from build123d import *

# Parameters (mm, degrees)
BOSS_EXTRUDE1_DEPTH = 25.4
SKETCH2_R           = 1.5875
BOSS_EXTRUDE2_DEPTH = 3.175


with BuildPart() as part:
    # Sketch1 → Boss-Extrude1 (new body)
    with BuildSketch(Plane(origin=(0, 0, 0), x_dir=(1, 0, 0), z_dir=(0, 1, 0))):
        with BuildLine():
            Line((-30.48, -31.75), (30.48, -31.75))
            ThreePointArc((30.48, -31.75), (35.868153673, -29.518153673), (38.1, -24.13))
            Line((38.1, -24.13), (38.1, 24.13))
            ThreePointArc((38.1, 24.13), (35.868153673, 29.518153673), (30.48, 31.75))
            Line((30.48, 31.75), (-30.48, 31.75))
            ThreePointArc((-30.48, 31.75), (-35.868153673, 29.518153673), (-38.1, 24.13))
            Line((-38.1, 24.13), (-38.1, -24.13))
            ThreePointArc((-38.1, -24.13), (-35.868153673, -29.518153673), (-30.48, -31.75))
        make_face()
    extrude(amount=BOSS_EXTRUDE1_DEPTH)

    # Sketch2 → Boss-Extrude2 (add)
    # profile 1 of 2: a face of its own
    with BuildSketch(Plane(origin=(0, 0, 0), x_dir=(1, 0, 0), z_dir=(0, 1, 0))):
        with BuildLine():
            Line((-24.869490834, -31.75), (24.869490834, -31.75))
            Line((24.869490834, -31.75), (24.869490834, -36.754911613))
            ThreePointArc((24.869490834, -36.754911613), (24.125542058, -38.550962837), (22.329490834, -39.294911613))
            Line((22.329490834, -39.294911613), (-22.329490834, -39.294911613))
            ThreePointArc((-22.329490834, -39.294911613), (-24.125542058, -38.550962837), (-24.869490834, -36.754911613))
            Line((-24.869490834, -36.754911613), (-24.869490834, -31.75))
        make_face()
        with Locations(Location((12.7, -35.71875, 0), (0, 0, 270))):
            Circle(SKETCH2_R, mode=Mode.SUBTRACT)
        with Locations(Location((-12.7, -35.71875, 0), (0, 0, 90))):
            Circle(SKETCH2_R, mode=Mode.SUBTRACT)
    # profile 2 of 2: a face of its own
    with BuildSketch(Plane(origin=(0, 0, 0), x_dir=(1, 0, 0), z_dir=(0, 1, 0))):
        with BuildLine():
            Line((-24.869490834, 31.75), (-24.869490834, 36.754911613))
            ThreePointArc((-24.869490834, 36.754911613), (-24.125542058, 38.550962837), (-22.329490834, 39.294911613))
            Line((-22.329490834, 39.294911613), (22.329490834, 39.294911613))
            ThreePointArc((22.329490834, 39.294911613), (24.125542058, 38.550962837), (24.869490834, 36.754911613))
            Line((24.869490834, 36.754911613), (24.869490834, 31.75))
            Line((24.869490834, 31.75), (-24.869490834, 31.75))
        make_face()
        with Locations(Location((12.7, 35.71875, 0), (0, 0, 90))):
            Circle(SKETCH2_R, mode=Mode.SUBTRACT)
        with Locations(Location((-12.7, 35.71875, 0), (0, 0, 270))):
            Circle(SKETCH2_R, mode=Mode.SUBTRACT)
    extrude(amount=BOSS_EXTRUDE2_DEPTH)


solid = part.part
Read the model definition and answer for the solid it produces. Units are mm, in the model's axes. A direction names the side the tool comes from. Give positions to 0.01 mm unless a question says otherwise; leave off trailing zeros. Loops run counter-clockwise (first coordinate to the right, second up) from the corner with the lowest first, then second, coordinate; pieces in that order, holes last. Notation, with made-up numbers: (36, 52) - (44, 52) arc R22 ccw to (44, 68) - close; hole circle Ø2 at (29.5, 33.5). An arc over 180 degrees is marked (long way). Answer as CSV lines item,"result". Start each with the question number.
1) Find section B-B (y = 24). Write down the section's boundary in (x, z), then the cut area to 3 significant figures.
2) Find section A-A (x = 12.7). Write down the section's boundary in (y, z) (3 decimals), then the cut area to 3 significant figures.
3) Find section C-C (x = 23.5). Write down the section's boundary in (y, z) (3 decimals).
4) Determine the mould class of faces 5 (the face through (35.927, 12.522, -29.459)), 6 (the face through (-1, 25.4, 0)), 7 (the face through (-13.177, 1.565, 34.205)) for opening direction X: released by +X, released by -X, zero draft, split by the parting line, or undercut.
5) Which of the six approach directions +Z, -Z, +X, -X, +Y, -Y give full straight-line access (tool end or side, diameter ignored) to faces 1 (the face through (24.869, 2, -34)), 2 (the face through (0, 3.175, -36)), 3 (the face through (0, 2, -39.295)), 4 (the face through (24.869, 2, 34))?
6) Straight lines are drawn through the part: L1, parallel to Z at x = 17.5, y = 4.5; L2, parallel to X at y = 3.25, z = -29. For each, find the intervals that lie inside material, in ascending order. Write a range as from..to.
7) Each of these flat-tipped pins is pushed along its axis until it touches: pin 1 Ø1 at (y, z) = (2.5, -35) entering from -X; pin 2 Ø10 at (x, y) = (21.5, 13) entering from +Z; pin 3 Ø6 at (x, z) = (12, 37) entering from +Y (3 decimals). Where does it stop, or does it pass through?
Findings below:
1,outline,"(-38.1, -24.13) arc R7.62 ccw to (-30.48, -31.75) - (30.48, -31.75) arc R7.62 ccw to (38.1, -24.13) - (38.1, 24.13) arc R7.62 ccw to (30.48, 31.75) - (-30.48, 31.75) arc R7.62 ccw to (-38.1, 24.13) - close"
1,area,"4,790 mm^2"
2,outline,"(0, -39.295) - (3.175, -39.295) - (3.175, -37.306) - (0, -37.306) - close; (0, -34.131) - (3.175, -34.131) - (3.175, -31.75) - (25.4, -31.75) - (25.4, 31.75) - (3.175, 31.75) - (3.175, 34.131) - (0, 34.131) - close; (0, 37.306) - (3.175, 37.306) - (3.175, 39.295) - (0, 39.295) - close"
2,area,"1,640 mm^2"
3,outline,"(0, -39.009) - (3.175, -39.009) - (3.175, -31.75) - (25.4, -31.75) - (25.4, 31.75) - (3.175, 31.75) - (3.175, 39.009) - (0, 39.009) - close"
4,face 5,"released by +X"
4,face 6,"zero draft"
4,face 7,"undercut"
5,face 1,"-Z, +X, +Y, -Y"
5,face 2,"-Z, +X, -X, +Y"
5,face 3,"-Z, +X, -X, +Y, -Y"
5,face 4,"+Z, +X, +Y, -Y"
6,L1,"-31.75..31.75"
6,L2,"-36.34..36.34"
7,pin 1,"x = -24.87"
7,pin 2,"z = 31.75"
7,pin 3,"y = 3.175"
